For this review, take the finished solid that the model builds, in its own axes (mm). Face numbers are marked on the shaded views. A direction names the side the tool comes from. Coordinates: 2 decimals unless noted, no trailing zeros. Order: outer loops, then holes, each group sorted by start corner. A loop starts at its lowest first (then second) coordinate and runs counter-clockwise, first axis right, second up. Notation, with made-up numbers: M 70,-21 L 116,-21 A8 cw 116,-13 Z; hole C 89.5,48.5 d4. An arc over 180 degrees is marked long. Use CSV: the item, a comma, the result in double quotes.
```python
from build123d import *

# Parameters (mm, degrees)
BOSS_EXTRUDE1_DEPTH      = 8.4
BOSS_EXTRUDE1_DEPTH_BACK = 8.4
FILLET1_R                = 6
CUT_EXTRUDE2_DEPTH       = 10
CUT_EXTRUDE1_DEPTH       = 10
CUT_EXTRUDE1_DEPTH_BACK  = 10
SKETCH3_W                = 1
SKETCH3_H                = 7.737404144
SKETCH5_R                = 1.5
CUT_EXTRUDE3_DEPTH       = 7
SKETCH6_W                = 1.82
SKETCH6_H                = 29.05
CUT_EXTRUDE4_DEPTH       = 7


with BuildPart() as part:
    # Sketch1 → Boss-Extrude1 (new, two sides: drawn at the far end of the back side and taken through both)
    with BuildSketch(Plane.XY.offset(-BOSS_EXTRUDE1_DEPTH_BACK)):
        Polygon((0, 0), (0, 36), (3.175, 36), (3.175, 3.175), (30, 3.175), (30, 0), align=None)
    extrude(amount=BOSS_EXTRUDE1_DEPTH + BOSS_EXTRUDE1_DEPTH_BACK)

    # Fillet1
    fillet1_edges = [part.edges().sort_by_distance(p)[0] for p in [
        (3.175, 3.175, 0),
    ]]
    fillet(fillet1_edges, radius=FILLET1_R)

    # Sketch4 → Cut-Extrude2 (cut)
    with BuildSketch(Plane.ZY):
        with BuildLine():
            Line((2.4, 31.225), (2.4, 29.725))
            ThreePointArc((2.4, 29.725), (0.9, 28.225), (-0.6, 29.725))
            Line((-0.6, 29.725), (-0.6, 31.225))
            ThreePointArc((-0.6, 31.225), (0.9, 32.725), (2.4, 31.225))
        make_face()
        with BuildLine():
            Line((-0.6, 9.725), (-0.6, 11.225))
            ThreePointArc((-0.6, 11.225), (0.9, 12.725), (2.4, 11.225))
            Line((2.4, 11.225), (2.4, 9.725))
            ThreePointArc((2.4, 9.725), (0.9, 8.225), (-0.6, 9.725))
        make_face()
    extrude(amount=-CUT_EXTRUDE2_DEPTH, mode=Mode.SUBTRACT)

    # Sketch3 → Cut-Extrude1 (cut, two sides: drawn at the far end of the back side and taken through both)
    with BuildSketch(Plane.XY.offset(-CUT_EXTRUDE1_DEPTH_BACK)):
        with Locations((3.675, 10.868702072)):
            Rectangle(SKETCH3_W, SKETCH3_H)
    extrude(amount=CUT_EXTRUDE1_DEPTH + CUT_EXTRUDE1_DEPTH_BACK, mode=Mode.SUBTRACT)

    # Sketch5 → Cut-Extrude3 (cut)
    with BuildSketch(Plane.XZ):
        with Locations(Location((19.41, 0.6, 0), (0, 0, 270))):
            Circle(SKETCH5_R)
        with Locations(Location((19.41, -5, 0), (0, 0, 270))):
            Circle(SKETCH5_R)
    extrude(amount=-CUT_EXTRUDE3_DEPTH, mode=Mode.SUBTRACT)

    # Sketch6 → Cut-Extrude4 (cut)
    with BuildSketch(Plane.ZY):
        with Locations((7.49, 21.475)):
            Rectangle(SKETCH6_W, SKETCH6_H)
    extrude(amount=-CUT_EXTRUDE4_DEPTH, mode=Mode.SUBTRACT)


solid = part.part
```
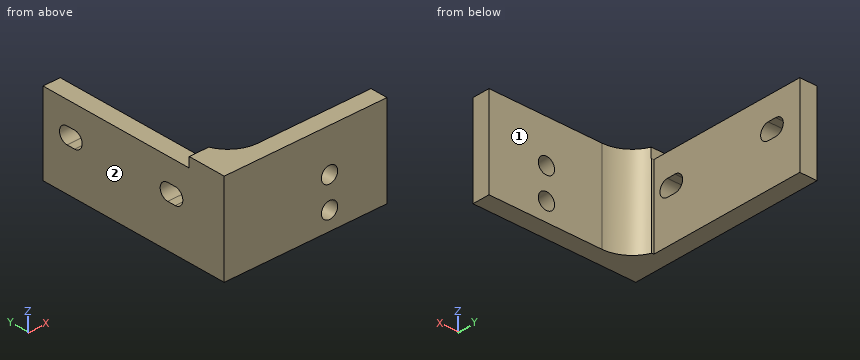
Item 1: For the marked faces 1 and 2, list the 3-axis set-ups (+Z, -Z, +X, -X, +Y, -Y) from which the entire face can be reached by the end or side of a thin tool; tool diameter is ignored.
Solutions:
face 1,"+Z, -Z, +X, +Y"
face 2,"+Z, -Z, -X, +Y, -Y"
Item 2: Add section A-A on y = 10.5. State the section outline as (x, z) points (3 decimals), and give its area (3 significant figures).
Solutions:
outline,"M 0,-8.4 L 3.175,-8.4 L 3.175,-0.6 L 0,-0.6 Z; M 0,2.4 L 3.175,2.4 L 3.175,6.58 L 0,6.58 Z"
area,"38.0 mm^2"
Item 3: To check wall thickness, follow line 1 along X through (y, z) = (0.9, 0.6); line 2 along Y through (x, z) = (3.25, -6.5); line 3 along Y through (x, z) = (13.25, -5) (3 decimals). State the ranges of each line that lie inside material, in increasing order. Write a range as [from, to].
Solutions:
line 1,"[0, 17.91], [20.91, 30]"
line 2,"[0, 7]"
line 3,"[0, 3.175]"
Item 4: Add section B-B on z = -5. State the section outline as (x, y) points (3 decimals).
Solutions:
outline,"M 0,0 L 17.91,0 L 17.91,3.175 L 9.175,3.175 A6 cw 3.583,7 L 3.175,7 L 3.175,36 L 0,36 Z; M 20.91,0 L 30,0 L 30,3.175 L 20.91,3.175 Z"
Item 5: Add section D-D on z = 0.6. State the section outline as (x, y) points (3 decimals), and give its area (3 significant figures).
Solutions:
outline,"M 0,0 L 17.91,0 L 17.91,3.175 L 9.175,3.175 A6 cw 3.583,7 L 3.175,7 L 3.175,8.255 L 0,8.255 Z; M 0,12.695 L 3.175,12.695 L 3.175,28.255 L 0,28.255 Z; M 0,32.695 L 3.175,32.695 L 3.175,36 L 0,36 Z; M 20.91,0 L 30,0 L 30,3.175 L 20.91,3.175 Z"
area,"169 mm^2"
Item 6: Add section C-C on x = 19.41. State the section outline as (y, z) points (3 decimals), and give its area (3 significant figures).
Solutions:
outline,"M 0,-8.4 L 3.175,-8.4 L 3.175,-6.5 L 0,-6.5 Z; M 0,-3.5 L 3.175,-3.5 L 3.175,-0.9 L 0,-0.9 Z; M 0,2.1 L 3.175,2.1 L 3.175,8.4 L 0,8.4 Z"
area,"34.3 mm^2"
Item 7: Clearance check with flat-ended pins moving along their axes: pin 1 Ø1.5 at (x, z) = (1.5, 7) entering from +Y; pin 2 Ø3.5 at (x, z) = (19.41, 0.6) entering from +Y (3 decimals); pin 3 Ø1.5 at (y, z) = (7.5, -2.5) entering from +X; pin 4 Ø5 at (x, y) = (19, 7.5) entering from -Z. State where each tip first meets the part, or that it passes through.
Solutions:
pin 1,"y = 36"
pin 2,"y = 3.175"
pin 3,"x = 3.69"
pin 4,"through"
